For this review, take the finished solid that the model builds, in its own axes (mm). Face numbers are marked on the shaded views. A direction names the side the tool comes from. Coordinates: 2 decimals unless noted, no trailing zeros. Loops run counter-clockwise (first coordinate to the right, second up) from the corner with the lowest first, then second, coordinate; pieces in that order, holes last. Notation, with made-up numbers: (15, -33) - (47, -33) arc R28 ccw to (47, -7) - close; hole circle Ø8 at (31, 80.5). An arc over 180 degrees is marked (long way). One line per item, written item: value. Start each with the question number.
1. Take a section at B-B, the plane x = 0. State the section outline as (y, z) points, and give its area (3 significant figures).
2. Take a section at C-C, the plane y = 0.75. State the section outline as (x, z) points, and give its area (3 significant figures).
3. Take a section at A-A, the plane z = 0. State the section outline as (x, y) points.
4. For the marked faces 3, 4 and 5, list the 3-axis set-ups (+Z, -Z, +X, -X, +Y, -Y) from which the entire face can be reached by the end or side of a thin tool; tool diameter is ignored.
5. Take a section at D-D, the plane z = 1.5. State the section outline as (x, y) points, and give its area (3 significant figures).
6. The part is to be moulded in two halves that separate along X. For the marked faces 1 and 2, say which applies: released by +X, released by -X, zero draft, split by the parting line, or undercut.
7. Insertion check: pin 1 (2 mm diameter, centred on x = 17, y = 2, fed in from -Z). The pin has a flat end and moves straight along its axis. Give the tip position at first contact, or say it passes through.
8. To check wall thickness, follow line 1 (X direction, y = 1.85, z = 0); line 2 (X direction, y = 3.35, z = -1.75); line 3 (Z direction, x = 17, y = 3.5). State the ranges of each line that lie inside material, in increasing order. Write a range as from..to.
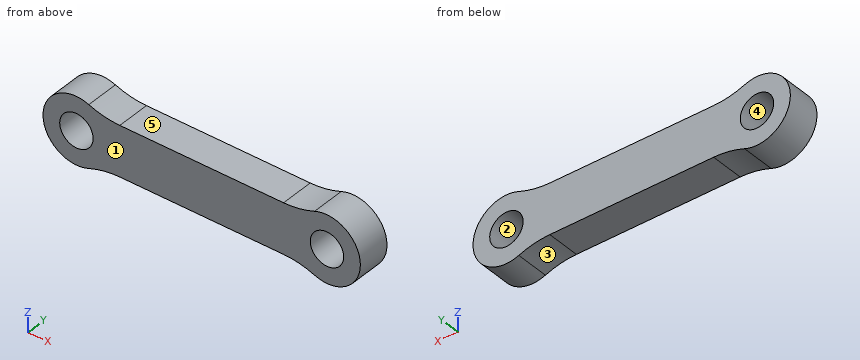
```python
from build123d import *

# Parameters (mm, degrees)
ESQUISSE1_R        = 2
BOSS_EXTRU_1_DEPTH = 4
CONG_1_R           = 10


with BuildPart() as part:
    # Esquisse1 → Boss.-Extru.1 (new body)
    with BuildSketch(Plane(origin=(0, 0, 0), x_dir=(1, 0, 0), z_dir=(0, 1, 0))):
        with BuildLine():
            Line((2.645751311, 3), (27.354248689, 3))
            ThreePointArc((27.354248689, 3), (34, 0), (27.354248689, -3))
            Line((27.354248689, -3), (2.645751311, -3))
            ThreePointArc((2.645751311, -3), (-4, 0), (2.645751311, 3))
        make_face()
        with Locations(Location((0, 0, 0), (0, 0, 270))):
            Circle(ESQUISSE1_R, mode=Mode.SUBTRACT)
        with Locations(Location((30, 0, 0), (0, 0, 270))):
            Circle(ESQUISSE1_R, mode=Mode.SUBTRACT)
    extrude(amount=BOSS_EXTRU_1_DEPTH)

    # Congé1
    cong_1_edges = [part.edges().sort_by_distance(p)[0] for p in [
        (2.645751311, 2, -3),
        (27.354248689, 2, -3),
        (27.354248689, 2, 3),
        (2.645751311, 2, 3),
    ]]
    fillet(cong_1_edges, radius=CONG_1_R)


solid = part.part
```
Solutions:
1. outline: (0, -4) - (4, -4) - (4, -2) - (0, -2) - close; (0, 2) - (4, 2) - (4, 4) - (0, 4) - close
1. area: 16.0 mm2
2. outline: (1.48, -3.71) arc R10 cw to (5.2, -3) - (24.8, -3) arc R10 cw to (28.52, -3.71) arc R4 ccw (long way) to (28.52, 3.71) arc R10 cw to (24.8, 3) - (5.2, 3) arc R10 cw to (1.48, 3.71) arc R4 ccw (long way) to start; hole circle Ø4 at (0, 0); hole circle Ø4 at (30, 0)
2. area: 214 mm2
3. outline: (-4, 0) - (-2, 0) - (-2, 4) - (-4, 4) - close; (2, 0) - (28, 0) - (28, 4) - (2, 4) - close; (32, 0) - (34, 0) - (34, 4) - (32, 4) - close
4. face 3: -Z, +Y, -Y
4. face 4: +Y, -Y
4. face 5: +Z, +Y, -Y
5. outline: (-3.71, 0) - (-1.32, 0) - (-1.32, 4) - (-3.71, 4) - close; (1.32, 0) - (28.68, 0) - (28.68, 4) - (1.32, 4) - close; (31.32, 0) - (33.71, 0) - (33.71, 4) - (31.32, 4) - close
5. area: 128 mm2
6. face 1: zero draft
6. face 2: undercut
7. pin 1: z = -3
8. line 1: -4..-2, 2..28, 32..34
8. line 2: -3.6..-0.97, 0.97..29.03, 30.97..33.6
8. line 3: -3..3
